Print and shaded views of the part. All mm, measured from the part's lowest x, y and z. Round coordinates to 2 decimals unless told otherwise and drop trailing zeros. Loops run counter-clockwise (first coordinate to the right, second up) from the corner with the lowest first, then second, coordinate; pieces in that order, holes last. Notation, with made-up numbers: M 13.5,56 L 17.5,56 A25 cw 17.5,78 Z; hole C 51,57.25 d7. An arc over 180 degrees is marked long. One line per item, written item: value. Start each with the question number.
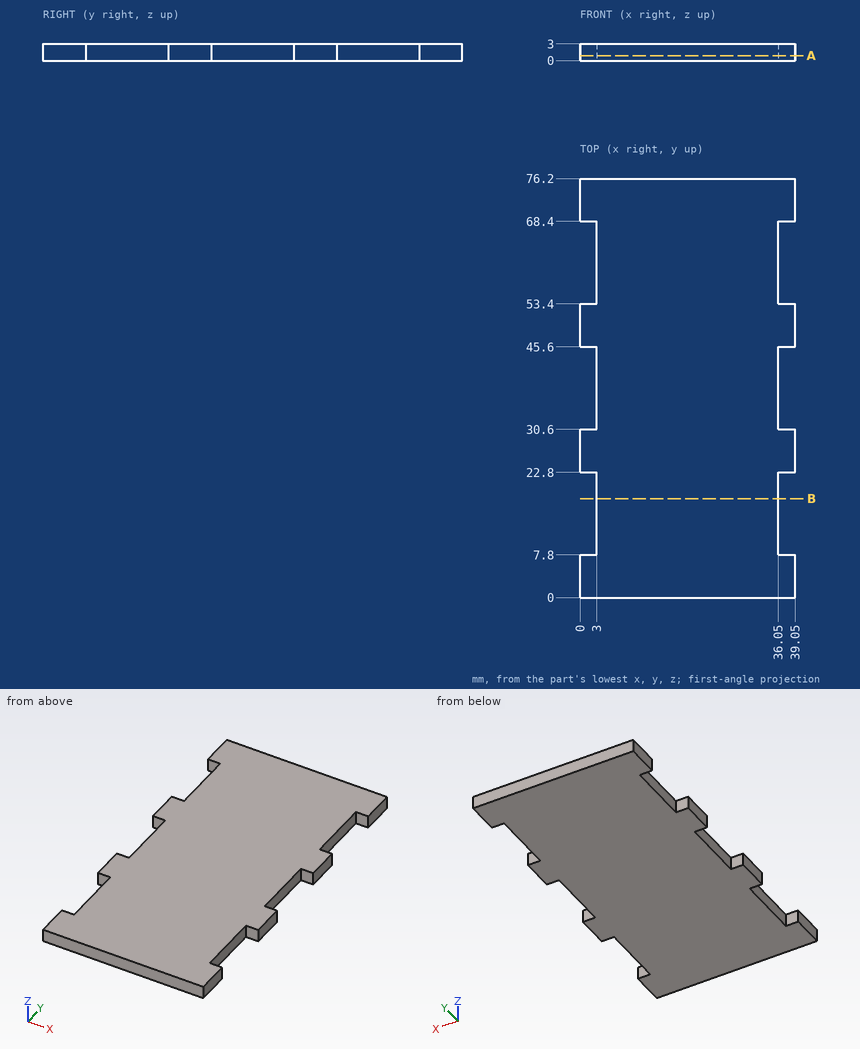
(1) Slice it at B-B, the plane y = 18. List the corners of the cut face in (x, z), and give its area (4 significant figures).
(2) Slice it at A-A, the plane z = 0.9. List the corners of the cut face in (x, y).
(3) Probe L1, parallel to Y at x = 37, z = 0.2; L2, parallel to X at y = 20, z = 2.65. List the from-to ranges inside material, lowest first.
(4) Flat gauge pins, fed straight in: P1, Ø2, axis at x = 26, y = 47, coming from the -Z side; P2, Ø0.9, axis at y = 61, z = 1.5, coming from the -X side. Where does each tip first touch, or does it go through?
Check result:
1. outline: M 3,0 L 36.05,0 L 36.05,3 L 3,3 Z
1. area: 99.15 mm^2
2. outline: M 0,0 L 39.05,0 L 39.05,7.8 L 36.05,7.8 L 36.05,22.8 L 39.05,22.8 L 39.05,30.6 L 36.05,30.6 L 36.05,45.6 L 39.05,45.6 L 39.05,53.4 L 36.05,53.4 L 36.05,68.4 L 39.05,68.4 L 39.05,76.2 L 0,76.2 L 0,68.4 L 3,68.4 L 3,53.4 L 0,53.4 L 0,45.6 L 3,45.6 L 3,30.6 L 0,30.6 L 0,22.8 L 3,22.8 L 3,7.8 L 0,7.8 Z
3. L1: y = 0 to 7.8, 22.8 to 30.6, 45.6 to 53.4, 68.4 to 76.2
3. L2: x = 3 to 36.05
4. P1: stops at z = 0
4. P2: stops at x = 3
